Can you work these out from the drawing? Everything is in mm from the part's minimum corner. Give positions to 0.01 mm unless a question says otherwise; leave off trailing zeros. Write each loop counter-clockwise with the first axis right and the second up, starting at its lowest first coordinate (ties: lowest second). Pieces come first, ordered by that corner, then holes. Notation, with made-up numbers: (59, 21.5) - (69, 21.5) arc R25 cw to (69, 44.5) - close; hole circle Ø10 at (79.25, 75.25). An arc over 180 degrees is marked (long way). Return JSON: item names as keys, results as strings. Group by question number.
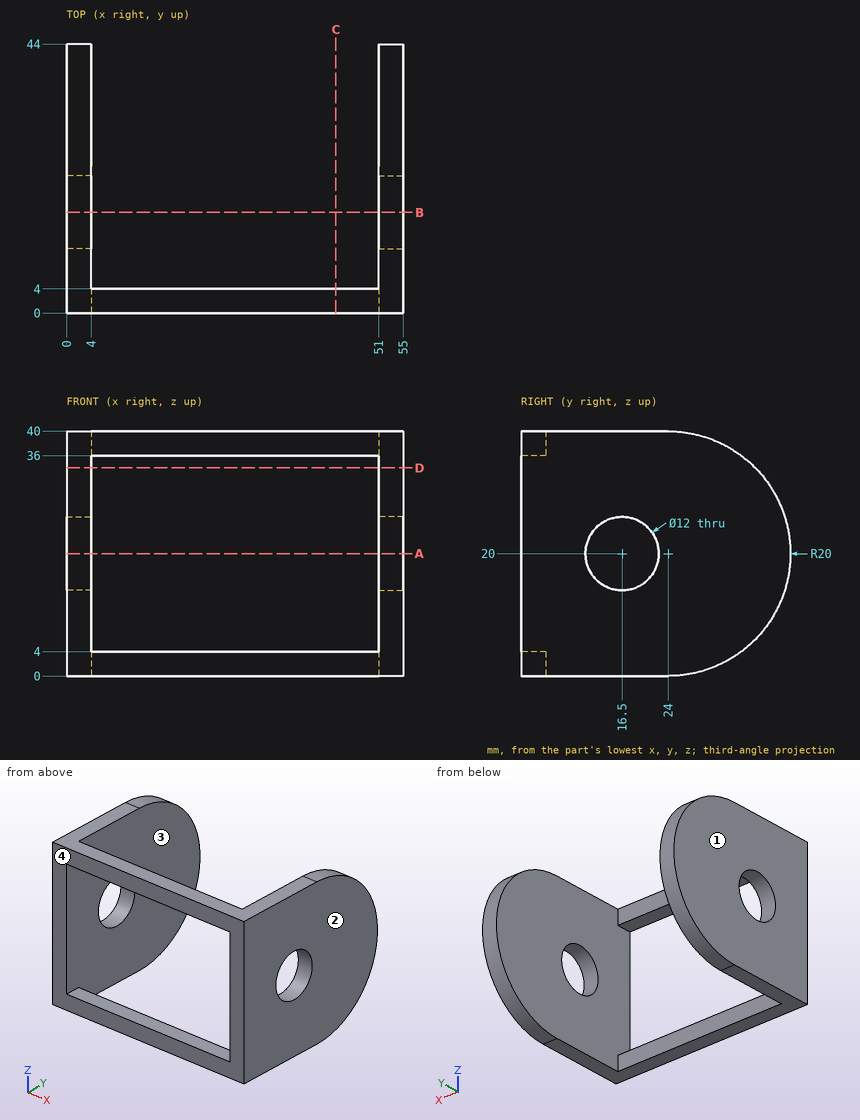
1) Imagine slicing it at D-D, the plane z = 34. Write out the boundary of the cut face in (x, y), and give its area (3 significant figures).
2) I need wall thicknesses on line 1 along Z through (x, y) = (29, 3.5); line 2 along X through (y, z) = (4, 33); line 3 along Y through (x, z) = (2.8, 20). Which ranges of each line are inside material? Lowest first, please.
3) Imagine slicing it at B-B, the plane y = 16.5. Write out the boundary of the cut face in (x, z).
4) Imagine slicing it at C-C, the plane x = 44. Write out the boundary of the cut face in (y, z).
5) Imagine slicing it at A-A, the plane z = 20. Write out the boundary of the cut face in (x, y), and give its area (3 significant figures).
6) Will these pins go through, and if not, where does the flat tip stop? pin 1 Ø5 at (y, z) = (14, 15.5) entering from -X; pin 2 Ø3 at (x, z) = (25.5, 38) entering from +Y.
7) We'd pull the mould along X, two halves only. Please class the marked faces 1, 2, 3 and 4: pulls with the +X half, pulls with the -X half, needs draft (parallel to the pull), parting line crosses it, or undercut.
Resolved:
{
 "1": {"outline": "(0, 0) - (4, 0) - (4, 38.28) - (0, 38.28) - close; (51, 0) - (55, 0) - (55, 38.28) - (51, 38.28) - close", "area": "306 mm^2"},
 "2": {"line 1": "0 to 4, 36 to 40", "line 2": "0 to 4, 51 to 55", "line 3": "0 to 10.5, 22.5 to 44"},
 "3": {"outline": "(0, 0) - (4, 0) - (4, 14) - (0, 14) - close; (0, 26) - (4, 26) - (4, 40) - (0, 40) - close; (51, 0) - (55, 0) - (55, 14) - (51, 14) - close; (51, 26) - (55, 26) - (55, 40) - (51, 40) - close"},
 "4": {"outline": "(0, 0) - (4, 0) - (4, 4) - (0, 4) - close; (0, 36) - (4, 36) - (4, 40) - (0, 40) - close"},
 "5": {"outline": "(0, 0) - (4, 0) - (4, 10.5) - (0, 10.5) - close; (0, 22.5) - (4, 22.5) - (4, 44) - (0, 44) - close; (51, 0) - (55, 0) - (55, 10.5) - (51, 10.5) - close; (51, 22.5) - (55, 22.5) - (55, 44) - (51, 44) - close", "area": "256 mm^2"},
 "6": {"pin 1": "x = 0", "pin 2": "y = 4"},
 "7": {"face 1": "pulls with the -X half", "face 2": "pulls with the +X half", "face 3": "undercut", "face 4": "needs draft"}
}
